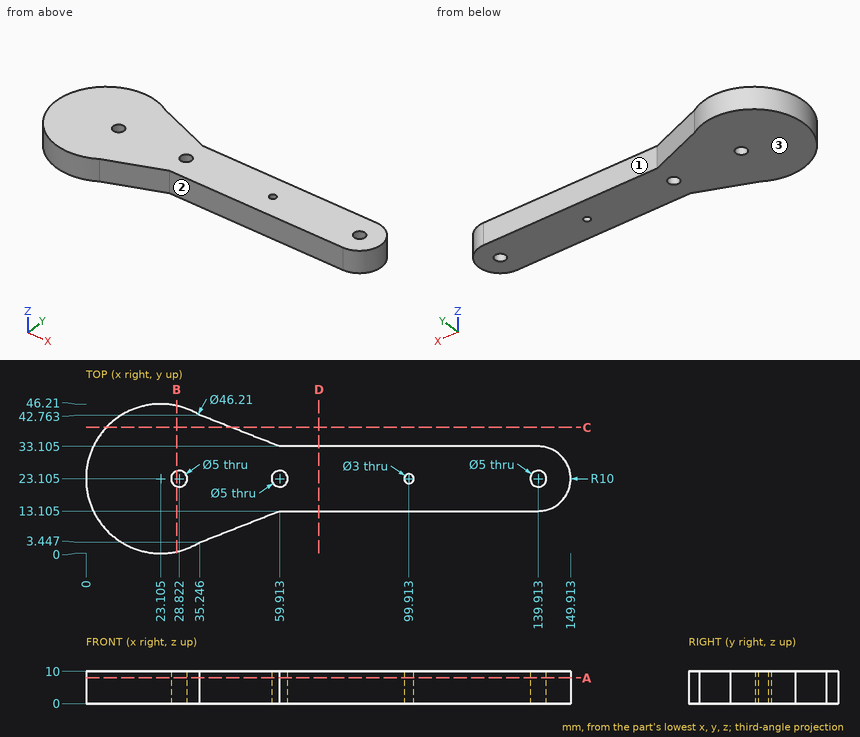
Check sheet for the drawn part. Datum: minimum x, y, z corner. Units: mm. A direction names the side the tool comes from. Round coordinates to 2 decimals unless told otherwise and drop trailing zeros. Order: outer loops, then holes, each group sorted by start corner. A loop starts at its lowest first (then second) coordinate and runs counter-clockwise, first axis right, second up.
(1) Access from +Z, -Z, +X, -X, +Y, -Y to the whole of each face (thin tool, end or side, straight path). Record for the marked faces 1, 2 and 3.
(2) Cross-section at B-B, the plane x = 28. Enter the section's corners in (y, z) (1 decimal).
(3) Scan lines: probe 1 along Y at (x, z) = (81, 9.5) (1 decimal); probe 2 along Y at (x, z) = (27, 1) (1 decimal); probe 3 along Y at (x, z) = (37, 8) (1 decimal). Record each from-to range of solid material in increasing order.
(4) Go/stop test with flat-tipped pins: P1, Ø3, axis at x = 20, z = 2, coming from the -Y side; P2, Ø3, axis at x = 15.5, z = 8, coming from the +Y side; P3, Ø6, axis at y = 41, z = 3, coming from the -X side. Record where each tip stops, or that it passes through.
(5) Cross-section at A-A, the plane z = 8. Enter the section's corners in (x, y) (1 decimal).
(6) Cross-section at D-D, the plane x = 72. Enter the section's corners in (y, z) (1 decimal).
(7) Cross-section at C-C, the plane y = 39. Enter the section's corners in (x, z).
Check sheet entries:
1. face 1: +Z, -Z, +X, +Y
1. face 2: +Z, -Z, +X, -Y
1. face 3: -Z, +X, -X, +Y, -Y
2. outline: (0.5, 0) - (20.7, 0) - (20.7, 10) - (0.5, 10) - close; (25.5, 0) - (45.7, 0) - (45.7, 10) - (25.5, 10) - close
3. probe 1: y = 13.1 to 33.1
3. probe 2: y = 0.3 to 21.4, 24.8 to 45.9
3. probe 3: y = 4.1 to 42.1
4. P1: stops at y = 0.06
4. P2: stops at y = 45.39
4. P3: stops at x = 5.44
5. outline: (35.2, 3.4) - (59.9, 13.1) - (139.9, 13.1) arc R10 ccw to (139.9, 33.1) - (59.9, 33.1) - (35.2, 42.8) arc R23.1 ccw (long way) to start; hole circle Ø5 at (28.8, 23.1); hole circle Ø5 at (59.9, 23.1); hole circle Ø3 at (99.9, 23.1); hole circle Ø5 at (139.9, 23.1)
6. outline: (13.1, 0) - (33.1, 0) - (33.1, 10) - (13.1, 10) - close
7. outline: (6.34, 0) - (44.86, 0) - (44.86, 10) - (6.34, 10) - close
